Design review of the part built by this model. Coordinates are the model's own, in mm. Give positions to 0.01 mm unless a question says otherwise; leave off trailing zeros. Loops run counter-clockwise (first coordinate to the right, second up) from the corner with the lowest first, then second, coordinate; pieces in that order, holes last. Notation, with made-up numbers: (50.5, 73) - (74.5, 73) arc R34 cw to (74.5, 103) - close; hole circle Ø6 at (9.5, 78). An arc over 180 degrees is marked (long way). Write each question's results on one line, items separated by ' | '.
from build123d import *

# Parameters (mm, degrees)
F0_R     = 88.9
F0_R_2   = 10.45593
F0_R_3   = 4
F1_DEPTH = 1
F4_DEPTH = 8
F3_R     = 88.9
F3_R_2   = 4
F5_DEPTH = 1


with BuildPart() as f1:
    # F0 (on Top) → F1 (new body)
    with BuildSketch(Plane.XY):
        Circle(F0_R)
        with BuildLine():
            ThreePointArc((-72.645684, -12.898561), (-70.900296, -6.361347), (-64.768881, -3.5))
            Line((-64.768881, -3.5), (-22.273598, -3.5))
            ThreePointArc((-22.273598, -3.5), (-18.966296, -4.493828), (-16.754625, -7.146081))
            ThreePointArc((-16.754625, -7.146081), (-12.879905, -12.879905), (-7.146081, -16.754625))
            ThreePointArc((-7.146081, -16.754625), (-4.493828, -18.966296), (-3.5, -22.273598))
            Line((-3.5, -22.273598), (-3.5, -64.768881))
            ThreePointArc((-3.5, -64.768881), (-6.361347, -70.900296), (-12.898561, -72.645684))
            ThreePointArc((-12.898561, -72.645684), (-52.17168, -52.17168), (-72.645684, -12.898561))
        make_face(mode=Mode.SUBTRACT)
        with BuildLine():
            ThreePointArc((72.645684, -12.898561), (52.17168, -52.17168), (12.898561, -72.645684))
            ThreePointArc((12.898561, -72.645684), (6.361347, -70.900296), (3.5, -64.768881))
            Line((3.5, -64.768881), (3.5, -22.273598))
            ThreePointArc((3.5, -22.273598), (4.493828, -18.966296), (7.146081, -16.754625))
            ThreePointArc((7.146081, -16.754625), (12.398278, -13.344161), (16.184999, -8.356418))
            ThreePointArc((16.184999, -8.356418), (18.300608, -6.043543), (21.29386, -5.113148))
            Line((21.29386, -5.113148), (64.768881, -3.5))
            ThreePointArc((64.768881, -3.5), (70.900296, -6.361347), (72.645684, -12.898561))
        make_face(mode=Mode.SUBTRACT)
        with BuildLine():
            ThreePointArc((-72.645684, 12.898561), (-52.17168, 52.17168), (-12.898561, 72.645684))
            ThreePointArc((-12.898561, 72.645684), (-6.361347, 70.900296), (-3.5, 64.768881))
            Line((-3.5, 64.768881), (-3.5, 22.273598))
            ThreePointArc((-3.5, 22.273598), (-4.493828, 18.966296), (-7.146081, 16.754625))
            ThreePointArc((-7.146081, 16.754625), (-12.879905, 12.879905), (-16.754625, 7.146081))
            ThreePointArc((-16.754625, 7.146081), (-18.966296, 4.493828), (-22.273598, 3.5))
            Line((-22.273598, 3.5), (-64.768881, 3.5))
            ThreePointArc((-64.768881, 3.5), (-70.900296, 6.361347), (-72.645684, 12.898561))
        make_face(mode=Mode.SUBTRACT)
        Circle(F0_R_2, mode=Mode.SUBTRACT)
        with BuildLine():
            Line((3.5, 22.273598), (3.5, 64.768881))
            ThreePointArc((3.5, 64.768881), (6.361347, 70.900296), (12.898561, 72.645684))
            ThreePointArc((12.898561, 72.645684), (52.17168, 52.17168), (72.645684, 12.898561))
            ThreePointArc((72.645684, 12.898561), (70.900296, 6.361347), (64.768881, 3.5))
            Line((64.768881, 3.5), (22.273598, 3.5))
            ThreePointArc((22.273598, 3.5), (18.966296, 4.493828), (16.754625, 7.146081))
            ThreePointArc((16.754625, 7.146081), (12.879905, 12.879905), (7.146081, 16.754625))
            ThreePointArc((7.146081, 16.754625), (4.493828, 18.966296), (3.5, 22.273598))
        make_face(mode=Mode.SUBTRACT)
        Circle(F0_R_2)
        Circle(F0_R_3, mode=Mode.SUBTRACT)
    extrude(amount=F1_DEPTH)

    # F0 (on Top) → F4 (join)
    with BuildSketch(Plane.XY):
        Circle(F0_R_2)
        Circle(F0_R_3, mode=Mode.SUBTRACT)
    extrude(amount=F4_DEPTH)

    # F3 (on offset) → F5 (join)
    with BuildSketch(Plane.XY.offset(7)):
        Circle(F3_R)
        with BuildLine():
            Line((-3.5, -22.273598), (-3.5, -64.768881))
            ThreePointArc((-3.5, -64.768881), (-6.361347, -70.900296), (-12.898561, -72.645684))
            ThreePointArc((-12.898561, -72.645684), (-52.17168, -52.17168), (-72.645684, -12.898561))
            ThreePointArc((-72.645684, -12.898561), (-70.900296, -6.361347), (-64.768881, -3.5))
            Line((-64.768881, -3.5), (-22.273598, -3.5))
            ThreePointArc((-22.273598, -3.5), (-18.966296, -4.493828), (-16.754625, -7.146081))
            ThreePointArc((-16.754625, -7.146081), (-12.879905, -12.879905), (-7.146081, -16.754625))
            ThreePointArc((-7.146081, -16.754625), (-4.493828, -18.966296), (-3.5, -22.273598))
        make_face(mode=Mode.SUBTRACT)
        with BuildLine():
            ThreePointArc((7.146081, -16.754625), (12.398278, -13.344161), (16.184999, -8.356418))
            ThreePointArc((16.184999, -8.356418), (18.300608, -6.043543), (21.29386, -5.113148))
            Line((21.29386, -5.113148), (64.768881, -3.5))
            ThreePointArc((64.768881, -3.5), (70.900296, -6.361347), (72.645684, -12.898561))
            ThreePointArc((72.645684, -12.898561), (52.17168, -52.17168), (12.898561, -72.645684))
            ThreePointArc((12.898561, -72.645684), (6.361347, -70.900296), (3.5, -64.768881))
            Line((3.5, -64.768881), (3.5, -22.273598))
            ThreePointArc((3.5, -22.273598), (4.493828, -18.966296), (7.146081, -16.754625))
        make_face(mode=Mode.SUBTRACT)
        with BuildLine():
            ThreePointArc((-7.146081, 16.754625), (-12.879905, 12.879905), (-16.754625, 7.146081))
            ThreePointArc((-16.754625, 7.146081), (-18.966296, 4.493828), (-22.273598, 3.5))
            Line((-22.273598, 3.5), (-64.768881, 3.5))
            ThreePointArc((-64.768881, 3.5), (-70.900296, 6.361347), (-72.645684, 12.898561))
            ThreePointArc((-72.645684, 12.898561), (-52.17168, 52.17168), (-12.898561, 72.645684))
            ThreePointArc((-12.898561, 72.645684), (-6.361347, 70.900296), (-3.5, 64.768881))
            Line((-3.5, 64.768881), (-3.5, 22.273598))
            ThreePointArc((-3.5, 22.273598), (-4.493828, 18.966296), (-7.146081, 16.754625))
        make_face(mode=Mode.SUBTRACT)
        Circle(F3_R_2, mode=Mode.SUBTRACT)
        with BuildLine():
            ThreePointArc((16.754625, 7.146081), (12.879905, 12.879905), (7.146081, 16.754625))
            ThreePointArc((7.146081, 16.754625), (4.493828, 18.966296), (3.5, 22.273598))
            Line((3.5, 22.273598), (3.5, 64.768881))
            ThreePointArc((3.5, 64.768881), (6.361347, 70.900296), (12.898561, 72.645684))
            ThreePointArc((12.898561, 72.645684), (52.17168, 52.17168), (72.645684, 12.898561))
            ThreePointArc((72.645684, 12.898561), (70.900296, 6.361347), (64.768881, 3.5))
            Line((64.768881, 3.5), (22.273598, 3.5))
            ThreePointArc((22.273598, 3.5), (18.966296, 4.493828), (16.754625, 7.146081))
        make_face(mode=Mode.SUBTRACT)
    extrude(amount=F5_DEPTH)


solid = f1.part
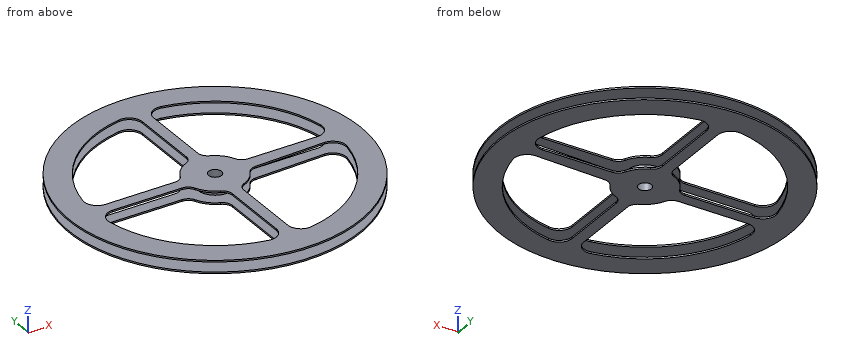
(1) Take a section at D-D on x = -28.5. Give the boundary of the cut face in (y, z).
Answers below:
outline: (-84.21, 0) - (-68.06, 0) - (-68.06, 1) - (-84.21, 1) - close; (-84.21, 7) - (-68.06, 7) - (-68.06, 8) - (-84.21, 8) - close; (-3.5, 0) - (3.5, 0) - (3.5, 1) - (-3.5, 1) - close; (-3.5, 7) - (3.5, 7) - (3.5, 8) - (-3.5, 8) - close; (68.06, 0) - (84.21, 0) - (84.21, 1) - (68.06, 1) - close; (68.06, 7) - (84.21, 7) - (84.21, 8) - (68.06, 8) - close
(2) Take a section at C-C on y = -53.5. Give the boundary of the cut face in (x, z), plus the area to 3 significant figures.
Answers below:
outline: (-71, 0) - (-50.81, 0) - (-50.81, 1) - (-71, 1) - close; (-71, 7) - (-50.81, 7) - (-50.81, 8) - (-71, 8) - close; (-3.5, 0) - (3.5, 0) - (3.5, 1) - (-3.5, 1) - close; (-3.5, 7) - (3.5, 7) - (3.5, 8) - (-3.5, 8) - close; (50.81, 0) - (71, 0) - (71, 1) - (50.81, 1) - close; (50.81, 7) - (71, 7) - (71, 8) - (50.81, 8) - close | area: 94.8 mm2
(3) Wall thickness on line 1 along Z through (x, y) = (-46.5, 66); line 2 along X through (y, z) = (68, 0.75); line 3 along Y through (x, z) = (0, 3.75): over which ranges is each line inside the solid? List them lowest first. Write a range as from..to.
Answers below:
line 1: 0..1, 7..8 | line 2: -57.26..-28.63, -4.18..4.18, 28.63..57.26 | line 3: -10.46..-4, 4..10.46
(4) Take a section at A-A on x = 0. Give the boundary of the cut face in (y, z), plus the area to 3 significant figures.
Answers below:
outline: (-88.9, 0) - (-4, 0) - (-4, 8) - (-88.9, 8) - (-88.9, 7) - (-10.46, 7) - (-10.46, 1) - (-88.9, 1) - close; (4, 0) - (88.9, 0) - (88.9, 1) - (10.46, 1) - (10.46, 7) - (88.9, 7) - (88.9, 8) - (4, 8) - close | area: 417 mm2
(5) Insertion check: P1, Ø1.1, axis at x = -40.5, z = 0.5, coming from the +Y side; P2, Ø0.5, axis at x = -46.5, z = 0.5, coming from the -Y side; P3, Ø0.8, axis at y = -38.5, z = 0.5, coming from the -X side; P4, Ø5, axis at x = 0, y = 0, coming from the -Z side. Each pin has a flat end and moves straight along its axis. Give the tip position at first contact, or say it passes through.
Answers below:
P1: y = 79.42 | P2: y = -75.92 | P3: x = -80.32 | P4: through
